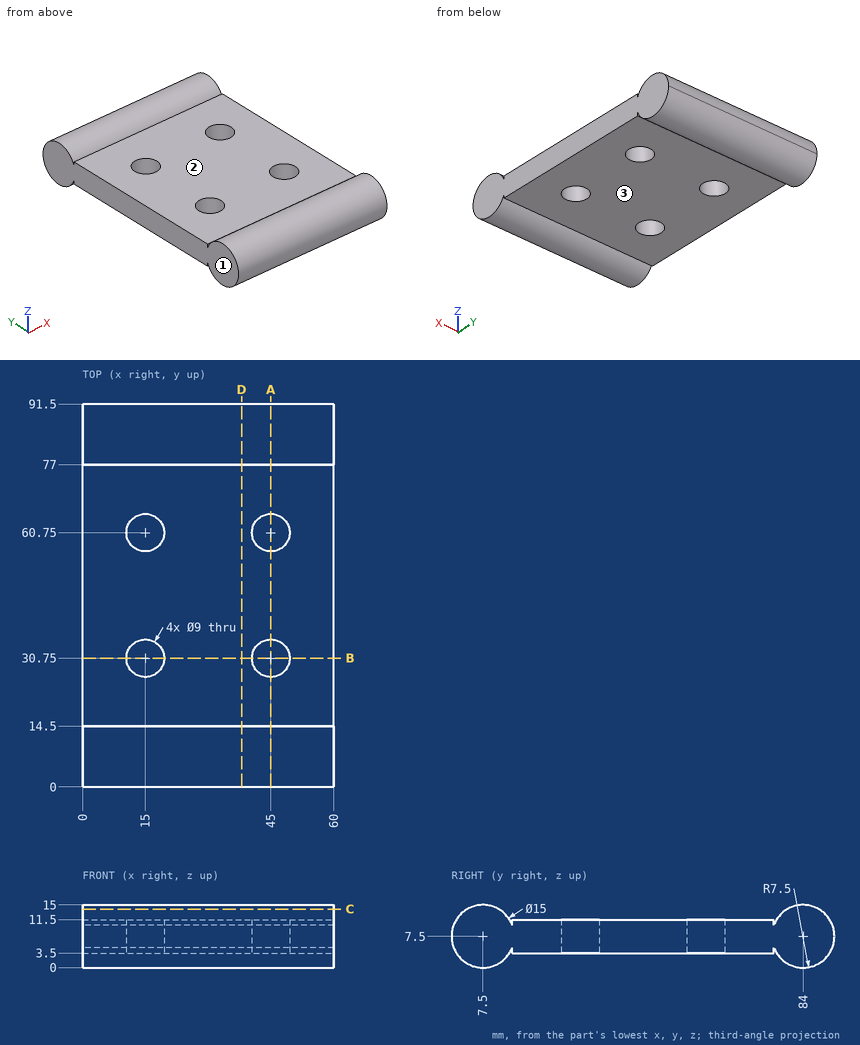
Design review of the part shown in the three views and the two pictorial views. Dimensions are in mm from the part's minimum x, y and z. A direction names the side the tool comes from. Give positions to 0.01 mm unless a question says otherwise; leave off trailing zeros. Write each loop counter-clockwise with the first axis right and the second up, starting at its lowest first coordinate (ties: lowest second). Pieces come first, ordered by that corner, then holes. Notation, with made-up numbers: (83, -17) - (141, -17) arc R12 ccw to (141, -12) - close; hole circle Ø3 at (50, 55). An arc over 180 degrees is marked (long way). Return JSON: item names as keys, results as strings. Group by question number.
(1) We need section C-C, the plane z = 14. Give the boundary of the cut face in (x, y), then the cut area to 3 significant figures.
(2) Insertion check: pin 1 (18 mm diameter, centred on x = 25, y = 59.5, fed in from +Z); pin 2 (3 mm diameter, centred on x = 23.5, z = 4, fed in from +Y); pin 3 (1.4 mm diameter, centred on x = 29.5, z = 4, fed in from +Y). Each pin has a flat end and moves straight along its axis. Give the tip position at first contact, or say it passes through.
(3) Machinability: for the marked faces 1, 2 and 3, which of the approach directions +Z, -Z, +X, -X, +Y, -Y give a long, thin tool a straight path to every point of the face, cutting with its end or side? Answer none if there is none.
(4) We need section D-D, the plane x = 38. Give the boundary of the cut face in (y, z), then the cut area to 3 significant figures.
(5) To check wall thickness, follow probe 1 along X at (y, z) = (31, 11.25); probe 2 along Y at (x, z) = (45, 8); probe 3 along Y at (x, z) = (45, 6.5). State the ranges of each line that lie inside material, in increasing order.
(6) We need section A-A, the plane x = 45. Give the boundary of the cut face in (y, z), then the cut area to 3 significant figures.
(7) We need section B-B, the plane y = 30.75. Give the boundary of the cut face in (x, z), then the cut area to 3 significant figures.
Reported:
{
 "1": {"outline": "(0, 3.76) - (60, 3.76) - (60, 11.24) - (0, 11.24) - close; (0, 80.26) - (60, 80.26) - (60, 87.74) - (0, 87.74) - close", "area": "898 mm2"},
 "2": {"pin 1": "stops at z = 11.5", "pin 2": "stops at y = 91.23", "pin 3": "stops at y = 90.96"},
 "3": {"face 1": "+Z, -Z, -X, +Y, -Y", "face 2": "+Z, +X, -X", "face 3": "-Z, +X, -X"},
 "4": {"outline": "(14.5, 3.5) - (77, 3.5) - (77, 4.81) arc R7.5 ccw (long way) to (77, 10.19) - (77, 11.5) - (14.5, 11.5) - (14.5, 10.19) arc R7.5 ccw (long way) to (14.5, 4.81) - close", "area": "850 mm2"},
 "5": {"probe 1": "x = 0 to 10.51, 19.49 to 40.51, 49.49 to 60", "probe 2": "y = 0.02 to 26.25, 35.25 to 56.25, 65.25 to 91.48", "probe 3": "y = 0.07 to 26.25, 35.25 to 56.25, 65.25 to 91.43"},
 "6": {"outline": "(14.5, 3.5) - (26.25, 3.5) - (26.25, 11.5) - (14.5, 11.5) - (14.5, 10.19) arc R7.5 ccw (long way) to (14.5, 4.81) - close; (35.25, 3.5) - (56.25, 3.5) - (56.25, 11.5) - (35.25, 11.5) - close; (65.25, 3.5) - (77, 3.5) - (77, 4.81) arc R7.5 ccw (long way) to (77, 10.19) - (77, 11.5) - (65.25, 11.5) - close", "area": "706 mm2"},
 "7": {"outline": "(0, 3.5) - (10.5, 3.5) - (10.5, 11.5) - (0, 11.5) - close; (19.5, 3.5) - (40.5, 3.5) - (40.5, 11.5) - (19.5, 11.5) - close; (49.5, 3.5) - (60, 3.5) - (60, 11.5) - (49.5, 11.5) - close", "area": "336 mm2"}
}
